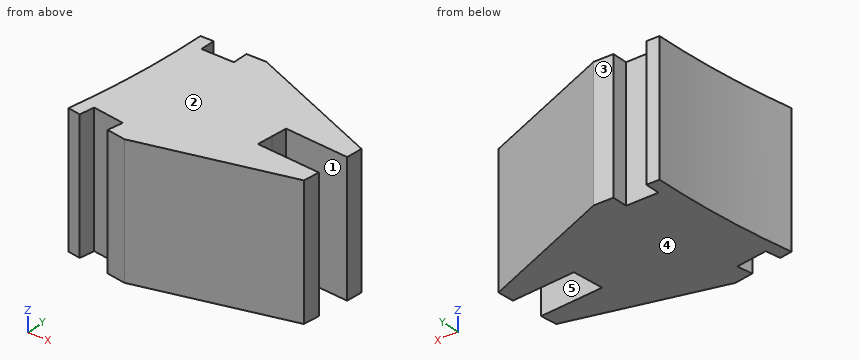
```python
from build123d import *

# Parameters (mm, degrees)
EXTRUDE_1_DEPTH     = 100
CUT_EXTRUDE_1_DEPTH = 849.335356313
CUT_EXTRUDE_2_DEPTH = 849.335356313
CUT_EXTRUDE_3_REACH = 850.335


with BuildPart() as part:
    # 草图1 → 凸台-拉伸1 (new body)
    with BuildSketch(Plane.XY):
        with BuildLine():
            Line((670, 0), (830, 0))
            ThreePointArc((830, 0), (826.841599416, -72.339266481), (817.390435, -144.127987464))
            Line((817.390435, -144.127987464), (659.821194518, -116.344279037))
            ThreePointArc((659.821194518, -116.344279037), (667.450447721, -58.394347641), (670, 0))
        make_face()
    extrude(amount=EXTRUDE_1_DEPTH)

    # 草图3 → 切除-拉伸1 (cut, through all)
    with BuildSketch(Plane.XY.offset(100)):
        with BuildLine():
            Line((778.121311296, -55.529045617), (777.031864512, -67.981479343))
            Line((777.031864512, -67.981479343), (775.942417727, -80.433913069))
            Line((775.942417727, -80.433913069), (825.658378988, -84.783496076))
            ThreePointArc((825.658378988, -84.783496076), (826.841599416, -72.339266481), (827.837272557, -59.878628624))
            Line((827.837272557, -59.878628624), (778.121311296, -55.529045617))
        make_face()
    extrude(amount=-CUT_EXTRUDE_1_DEPTH, mode=Mode.SUBTRACT)

    # 草图6 → 切除-拉伸2 (cut, through all)
    with BuildSketch(Plane(origin=(0, 0, 0), x_dir=(-1, 0, 0), z_dir=(0, 0, -1))):
        with BuildLine():
            Line((-669.669272048, -118.080760814), (-694.289465874, -122.421965255))
            ThreePointArc((-694.289465874, -122.421965255), (-695.331349084, -116.358562132), (-696.32028012, -110.286297853))
            Line((-696.32028012, -110.286297853), (-671.628071605, -106.375436227))
            ThreePointArc((-671.628071605, -106.375436227), (-670.674209045, -112.232371985), (-669.669272048, -118.080760814))
        make_face()
        with BuildLine():
            Line((-679.896432706, -11.867636377), (-704.892625085, -12.303946538))
            ThreePointArc((-704.892625085, -12.303946538), (-704.97315576, -6.152207526), (-705, 0))
            Line((-705, 0), (-680, 0))
            ThreePointArc((-680, 0), (-679.974107684, -5.934044139), (-679.896432706, -11.867636377))
        make_face()
    extrude(amount=-CUT_EXTRUDE_2_DEPTH, mode=Mode.SUBTRACT)

    # 草图7 → 切除-拉伸3 (cut, up to next)
    with BuildSketch(Plane.XY.offset(100), mode=Mode.PRIVATE) as cut_extrude_3_sk1:
        with BuildLine():
            Line((720, 0), (828.675083599, -46.878628624))
            ThreePointArc((828.675083599, -46.878628624), (829.668704781, -23.44867387), (830, 0))
            Line((830, 0), (720, 0))
        make_face()
    cut_extrude_3_tool1 = extrude(cut_extrude_3_sk1.sketch, amount=-CUT_EXTRUDE_3_REACH, mode=Mode.PRIVATE) & part.part
    # 草图7 → 切除-拉伸3 (cut, up to next)
    with BuildSketch(Plane.XY.offset(100), mode=Mode.PRIVATE) as cut_extrude_3_sk2:
        with BuildLine():
            Line((824.226035489, -97.731481226), (709.061582169, -125.02668792))
            Line((709.061582169, -125.02668792), (817.390435, -144.127987464))
            ThreePointArc((817.390435, -144.127987464), (821.135992387, -120.978022827), (824.226035489, -97.731481226))
        make_face()
    cut_extrude_3_tool2 = extrude(cut_extrude_3_sk2.sketch, amount=-CUT_EXTRUDE_3_REACH, mode=Mode.PRIVATE) & part.part
    add(cut_extrude_3_tool1.solids().sort_by_distance((793.038059, -15.657488, 100))[0], mode=Mode.SUBTRACT)
    add(cut_extrude_3_tool2.solids().sort_by_distance((783.708923, -122.289998, 100))[0], mode=Mode.SUBTRACT)


solid = part.part
```
CAD build for the part. Positions are in the model's coordinates, mm. Face numbers are marked on the shaded views. A direction names the side the tool comes from. Coordinates: 2 decimals unless noted, no trailing zeros. Order: outer loops, then holes, each group sorted by start corner. A loop starts at its lowest first (then second) coordinate and runs counter-clockwise, first axis right, second up. Notation, with made-up numbers: (22, 50) - (36, 50) arc R26 cw to (36, 64) - close; hole circle Ø2 at (47.5, 84). An arc over 180 degrees is marked (long way). Answer in a Markdown table with one row per item.
1. Flat gauge pins, fed straight in: P1, Ø8, axis at x = 714, y = -30.5, coming from the -Z side; P2, Ø3, axis at x = 722, z = 20, coming from the +Y side; P3, Ø1, axis at y = -103, z = 19.5, coming from the -X side; P4, Ø6, axis at x = 810.5, z = 79.5, coming from the -Y side. Where does each tip first touch, or does it go through?
Answer:
| item | result |
|---|---|
| P1 | z = 0 |
| P2 | y = -0.22 |
| P3 | x = 661.96 |
| P4 | y = -101.7 |
2. Slice it at A-A, the plane z = 62. List the corners of the cut face in (x, y).
Answer:
| item | result |
|---|---|
| outline | (659.82, -116.34) - (669.67, -118.08) arc R680 ccw to (671.63, -106.38) - (696.32, -110.29) arc R705 cw to (694.29, -122.42) - (709.06, -125.03) - (824.23, -97.73) arc R830 ccw to (825.66, -84.78) - (775.94, -80.43) - (778.12, -55.53) - (827.84, -59.88) arc R830 ccw to (828.68, -46.88) - (720, 0) - (705, 0) arc R705 cw to (704.89, -12.3) - (679.9, -11.87) arc R680 ccw to (680, 0) - (670, 0) arc R670 cw to start |
3. Slice it at C-C, the plane y = -42. List the corners of the cut face in (x, z), then the cut area to 3 significant figures.
Answer:
| item | result |
|---|---|
| outline | (668.68, 0) - (817.37, 0) - (817.37, 100) - (668.68, 100) - close |
| area | 14,900 mm² |
4. Pull direction Y, two halves, no side cores. Call the marked faces 3, 4 and 5: +Y half, -Y half, draft (parallel to the pull), parting line (faces both ways), or undercut.
Answer:
| item | result |
|---|---|
| face 3 | +Y half |
| face 4 | draft |
| face 5 | undercut |
5. Drill centre lines: L1, parallel to Y at x = 805, z = 66; L2, parallel to Y at x = 780, z = 70; L3, parallel to X at y = -4.5, z = 42.5. Where is each one in solid material? Low to high. Write a range as from..to.
Answer:
| item | result |
|---|---|
| L1 | -102.29..-82.98, -57.88..-36.67 |
| L2 | -108.21..-80.79, -55.69..-25.88 |
| L3 | 669.98..679.99, 704.99..730.43 |
6. 3-axis set-ups, long thin cutter, end or side, ignore diameter. For the marked faces 1 and 2: which of +Z, -Z, +X, -X, +Y, -Y reach the whole face in a straight line?
Answer:
| item | result |
|---|---|
| face 1 | +Z, -Z |
| face 2 | +Z, +X, -X, +Y, -Y |
7. Slice it at B-B, the plane x = 751. List the corners of the cut face in (y, z), then the cut area to 3 significant figures.
Answer:
| item | result |
|---|---|
| outline | (-115.09, 0) - (-13.37, 0) - (-13.37, 100) - (-115.09, 100) - close |
| area | 10,200 mm² |
